Design review of the part built by this model. Coordinates are the model's own, in mm. Give positions to 0.01 mm unless a question says otherwise; leave off trailing zeros. Loops run counter-clockwise (first coordinate to the right, second up) from the corner with the lowest first, then second, coordinate; pieces in that order, holes last.
from build123d import *

# Parameters (mm, degrees)
F1_DEPTH    = 9.525
F2_T1_DEPTH = 126.6954628883


# Not quite as in the source:
# - a fillet or chamfer that OpenCascade refuses, or shapes differently, is made with other operations: its cross-section is extruded or revolved along the edge and cut away or added


with BuildPart() as f1:
    # F0 (on Top) → F1 (new body)
    with BuildSketch(Plane.XY):
        Polygon((0, 76.5490606427), (0, 7.1380194277), (4.5535564423, 4.6766349114), (75.9337022901, 76.5490606427), align=None)
    extrude(amount=F1_DEPTH)

    # F2: fillet of radius 5.08 on 2 edges, made by hand

    # F2_s2 → F2_t1 (cut)
    with BuildSketch(Plane(origin=(-4.3499505247, -4.3799503673, 0), x_dir=(0, 0, 1), z_dir=(0.7046726854, 0.7095325267, 0))):
        with BuildLine():
            ThreePointArc((5.08, -0.0646004733), (1.4878975516, -1.5524980249), (0, -5.1446004733))
            Line((0, -5.1446004733), (0, -0.0646004733))
            Line((0, -0.0646004733), (5.08, -0.0646004733))
        make_face()
        with BuildLine():
            ThreePointArc((4.445, -0.0646004733), (8.0371024484, -1.5524980249), (9.525, -5.1446004733))
            Line((9.525, -5.1446004733), (9.525, -0.0646004733))
            Line((9.525, -0.0646004733), (4.445, -0.0646004733))
        make_face()
    extrude(amount=F2_T1_DEPTH, mode=Mode.SUBTRACT)


solid = f1.part
Q1. Take a section at A-A (z = 7). Give the boundary of the cut face in (x, y).
Results:
outline: (0, 7.14) - (3.92, 5.02) - (74.96, 76.55) - (0, 76.55) - close
Q2. Wall thickness on line 1 (X direction, y = 51.5, z = 4); line 2 (X direction, y = 14, z = 8); line 3 (Y direction, x = 11.5, z = 6.25): over which ranges is each line inside the solid? List them lowest first.
Results:
line 1: x = 0 to 50.89
line 2: x = 0 to 11.77
line 3: y = 12.14 to 76.55
Q3. Insertion check: pin 1 (2 mm diameter, centred on x = 33, y = 36, fed in from +Z); pin 2 (2 mm diameter, centred on x = 36, z = 8, fed in from -Y); pin 3 (1.5 mm diameter, centred on y = 31.5, z = 7, fed in from +X). Each pin has a flat end and moves straight along its axis. Give the tip position at first contact, or say it passes through.
Results:
pin 1: stops at z = 9.03
pin 2: stops at y = 36.87
pin 3: stops at x = 31.15
